The listing builds one solid part. Answer for the finished solid, in the listing's coordinates (mm). A direction names the side the tool comes from. Give positions to 0.01 mm unless a question says otherwise; leave off trailing zeros. Write each loop counter-clockwise with the first axis right and the second up, starting at its lowest first coordinate (ties: lowest second). Pieces come first, ordered by that corner, then holes. Notation, with made-up numbers: (10, -0.5) - (30, -0.5) arc R13 ccw to (30, 15.5) - close; hole circle Ø6 at (47, -2). An arc over 180 degrees is marked (long way). Answer as CSV lines item,"result". Start each with the question number.
(1) For faces 1 (the face through (-117.254, -708, 51)), 2 (the face through (-42.32, -708, 51)), determine the directions among +Z, -Z, +X, -X, +Y, -Y from which every point of the face is accessible in a straight line to the end or side of a thin tool.
(2) Straight lines are drawn through the part: probe 1 along Z at (x, y) = (-63.5, -895); probe 2 along X at (y, z) = (-876.5, 28). For each, find the intervals that lie inside material, in ascending order.
(3) Find section A-A (z = 31). Write down the section's boundary in (x, y).
(4) Find section B-B (y = -766.5). Write down the section's boundary in (x, z), then the cut area to 3 significant figures.
(5) Find section C-C (x = -86.5). Write down the section's boundary in (y, z), then the cut area to 3 significant figures.
(6) For a pull along Z with two mould halves and no side action, classify faces 3 (the face through (-115.991, -708, 52)), 4 (the face through (-80, -708, 89.575)), 5 (the face through (-41.054, -708, 51)) as pulls with the +Z half, pulls with the -Z half, needs draft (parallel to the pull), parting line crosses it, or undercut.
from build123d import *

# Parameters (mm, degrees)
F0_W     = 76.2
F0_H     = 76.2
F1_DEPTH = 609.6
F3_DEPTH = 914.4
F4_DEPTH = 304.8
F5_DEPTH = 508


with BuildPart() as f1:
    # F0 (on Front) → F1 (new body)
    with BuildSketch(Plane.XZ):
        with Locations((-79.1539917648, 51.4746750653)):
            Rectangle(F0_W, F0_H)
    extrude(amount=F1_DEPTH)

    # F2 (on face) → F3 (cut)
    with BuildSketch(Plane.XZ.offset(609.6)):
        Polygon((-42.3204526305, 88.3055701852), (-98.6881405115, 88.3055701852), (-115.9909814596, 88.3055701852), (-115.9909814596, 14.655277133), (-42.3204526305, 14.655277133), align=None)
    extrude(amount=-F3_DEPTH, mode=Mode.SUBTRACT)

    # F4 (add): a face of the model
    f4_faces = [f1.faces().sort_by_distance(p)[0] for p in [
        (-42.1316224993, -609.6, 51.4746750653),
    ]]
    extrude(f4_faces, amount=F4_DEPTH)

    # F5 (cut): a face of the model
    f5_faces = [f1.faces().sort_by_distance(p)[0] for p in [
        (-42.1316224993, 0, 51.4746750653),
    ]]
    extrude(f5_faces, amount=-F5_DEPTH, mode=Mode.SUBTRACT)


solid = f1.part
Result set:
1,face 1,"+Z, -Z, -X, +Y, -Y"
1,face 2,"+Y, -Y"
2,probe 1,"13.37 to 14.66, 88.31 to 89.57"
2,probe 2,"-117.25 to -115.99, -42.32 to -41.05"
3,outline,"(-117.25, -914.4) - (-115.99, -914.4) - (-115.99, -508) - (-117.25, -508) - close; (-42.32, -914.4) - (-41.05, -914.4) - (-41.05, -508) - (-42.32, -508) - close"
4,outline,"(-117.25, 13.37) - (-41.05, 13.37) - (-41.05, 89.57) - (-117.25, 89.57) - close; hole (-115.99, 14.66) - (-42.32, 14.66) - (-42.32, 88.31) - (-115.99, 88.31) - close"
4,area,"381 mm^2"
5,outline,"(-914.4, 13.37) - (-508, 13.37) - (-508, 14.66) - (-914.4, 14.66) - close; (-914.4, 88.31) - (-508, 88.31) - (-508, 89.57) - (-914.4, 89.57) - close"
5,area,"1,040 mm^2"
6,face 3,"undercut"
6,face 4,"pulls with the +Z half"
6,face 5,"needs draft"
